Read the model definition and answer for the solid it produces. Units are mm, in the model's axes. A direction names the side the tool comes from. Give positions to 0.01 mm unless a question says otherwise; leave off trailing zeros. Loops run counter-clockwise (first coordinate to the right, second up) from the corner with the lowest first, then second, coordinate; pieces in that order, holes last.
(1) Straight lines are drawn through the part: probe 1 along Y at (x, z) = (0, -10.8); probe 2 along Y at (x, z) = (52, -10); probe 3 along Z at (x, y) = (-52.5, -42). For each, find the intervals that lie inside material, in ascending order.
(2) Each of these flat-tipped pins is pushed along its axis until it touches: P1, Ø13.5, axis at x = 0, y = -45, coming from the -Z side; P2, Ø10, axis at x = 28, y = -45, coming from the +Z side; P3, Ø6, axis at x = 28.5, z = -8.5, coming from the +Y side; P4, Ø6, axis at x = -22.5, y = -79, coming from the -Z side. Where does it stop, or does it pass through?
(3) Find section A-A, the plane y = -45. Write down the section's boundary in (x, z).
(4) Find section D-D, the plane y = 31.5. Write down the section's boundary in (x, z).
(5) Find section B-B, the plane x = 28. Write down the section's boundary in (y, z).
(6) Which of the six approach directions +Z, -Z, +X, -X, +Y, -Y give full straight-line access (tool end or side, diameter ignored) to faces 5 (the face through (1, -77, -3)), 6 (the face through (0.896, -59.542, -4.714)), 7 (the face through (32.246, 44.813, -10.979))?
(7) Determine the mould class of faces 1 (the face through (59.944, -83.49, -1.521)), 2 (the face through (-51.524, -80.797, -1.479)), 3 (the face through (-54.76, -27.73, -10.98)), 4 (the face through (1, 1, -12.5)) for opening direction X: pulls with the +X half, pulls with the -X half, needs draft (parallel to the pull), parting line crosses it, or undercut.
(8) Find section C-C, the plane y = -2. Write down the section's boundary in (x, z), then the cut area to 3 significant figures.
```python
from build123d import *

# Parameters (mm, degrees)
EXTRUDE_1_DEPTH     = 64
CHAMFER_1_SIZE      = 8
SKETCH_4_R          = 4.25
CUT_EXTRUDE_1_DEPTH = 110.073337851
SKETCH_6_R          = 4.25
CUT_EXTRUDE_2_DEPTH = 10


with BuildPart() as part:
    # 草图1 → 凸台-拉伸1 (new, symmetric)
    with BuildSketch(Plane(origin=(0, 0, 0), x_dir=(0, 0, -1), z_dir=(1, 0, 0))):
        with BuildLine():
            Line((0, 87.434221161), (3, 87.434221161))
            Line((3, 87.434221161), (3, 66.740486184))
            ThreePointArc((3, 66.740486184), (3.565077878, 64.198514208), (5.153873841, 62.135346276))
            Line((5.153873841, 62.135346276), (10.346126159, 57.798874885))
            ThreePointArc((10.346126159, 57.798874885), (11.934922122, 55.735706953), (12.5, 53.193734977))
            Line((12.5, 53.193734977), (12.5, -53.193734977))
            ThreePointArc((12.5, -53.193734977), (11.934922122, -55.735706953), (10.346126159, -57.798874885))
            Line((10.346126159, -57.798874885), (5.153873841, -62.135346276))
            ThreePointArc((5.153873841, -62.135346276), (3.565077878, -64.198514208), (3, -66.740486184))
            Line((3, -66.740486184), (3, -87.434221161))
            Line((3, -87.434221161), (0, -87.434221161))
            Line((0, -87.434221161), (0, -66.285275099))
            ThreePointArc((0, -66.285275099), (0.565077878, -63.743303123), (2.153873841, -61.680135191))
            Line((2.153873841, -61.680135191), (7.346126159, -57.3436638))
            ThreePointArc((7.346126159, -57.3436638), (8.934922122, -55.280495868), (9.5, -52.738523893))
            Line((9.5, -52.738523893), (9.5, 52.738523893))
            ThreePointArc((9.5, 52.738523893), (8.934922122, 55.280495868), (7.346126159, 57.3436638))
            Line((7.346126159, 57.3436638), (2.153873841, 61.680135191))
            ThreePointArc((2.153873841, 61.680135191), (0.565077878, 63.743303123), (0, 66.285275099))
            Line((0, 66.285275099), (0, 87.434221161))
        make_face()
    extrude(amount=EXTRUDE_1_DEPTH, both=True)

    # 倒角1
    chamfer_1_edges = [part.edges().sort_by_distance(p)[0] for p in [
        (-64, 87.434221161, -1.5),
        (-64, -87.434221161, -1.5),
        (64, -87.434221161, -1.5),
        (64, 87.434221161, -1.5),
    ]]
    chamfer(chamfer_1_edges, length=CHAMFER_1_SIZE)

    # 草图4 → 切除-拉伸1 (cut, through all)
    with BuildSketch(Plane.XY):
        with Locations((-52.800881805, 76.743624005)):
            Circle(SKETCH_4_R)
        with Locations((53.199118195, 76.743624005)):
            Circle(SKETCH_4_R)
        with Locations((-52.800881805, 31.5)):
            Circle(SKETCH_4_R)
        with Locations((-28, 45)):
            Circle(SKETCH_4_R)
        with Locations((0, 45)):
            Circle(SKETCH_4_R)
        with Locations(Location((52.800881805, 31.5, 0), (0, 0, 180))):
            Circle(SKETCH_4_R)
        with Locations(Location((28, 45, 0), (0, 0, 180))):
            Circle(SKETCH_4_R)
        with Locations(Location((53.199118195, -76.743624005, 0), (0, 0, 270))):
            Circle(SKETCH_4_R)
        with Locations((52.800881805, -31.5)):
            Circle(SKETCH_4_R)
        with Locations((28, -45)):
            Circle(SKETCH_4_R)
        with Locations(Location((0, -45, 0), (0, 0, 180))):
            Circle(SKETCH_4_R)
        with Locations(Location((-28, -45, 0), (0, 0, 180))):
            Circle(SKETCH_4_R)
        with Locations(Location((-52.800881805, -31.5, 0), (0, 0, 180))):
            Circle(SKETCH_4_R)
        with Locations(Location((-52.800881805, -76.743624005, 0), (0, 0, 270))):
            Circle(SKETCH_4_R)
    extrude(amount=-CUT_EXTRUDE_1_DEPTH, mode=Mode.SUBTRACT)

    # 草图6 → 切除-拉伸2 (cut)
    with BuildSketch(Plane(origin=(0, 0, -12.5), x_dir=(-1, 0, 0), z_dir=(0, 0, -1))):
        with Locations((-53, 0)):
            Circle(SKETCH_6_R)
        with Locations((53, 0)):
            Circle(SKETCH_6_R)
    extrude(amount=-CUT_EXTRUDE_2_DEPTH, mode=Mode.SUBTRACT)


solid = part.part
```
Entries:
1. probe 1: y = -57.38 to -49.25, -40.75 to 40.75, 49.25 to 57.38
1. probe 2: y = -58.09 to -35.67, -27.33 to -4.13, 4.13 to 27.33, 35.67 to 58.09
1. probe 3: z = -12.5 to -9.5
2. P1: stops at z = -12.5
2. P2: stops at z = -9.5
2. P3: stops at y = 61.85
2. P4: stops at z = -3
3. outline: (-64, -12.5) - (-32.25, -12.5) - (-32.25, -9.5) - (-64, -9.5) - close; (-23.75, -12.5) - (-4.25, -12.5) - (-4.25, -9.5) - (-23.75, -9.5) - close; (4.25, -12.5) - (23.75, -12.5) - (23.75, -9.5) - (4.25, -9.5) - close; (32.25, -12.5) - (64, -12.5) - (64, -9.5) - (32.25, -9.5) - close
4. outline: (-64, -12.5) - (-57.05, -12.5) - (-57.05, -9.5) - (-64, -9.5) - close; (-48.55, -12.5) - (48.55, -12.5) - (48.55, -9.5) - (-48.55, -9.5) - close; (57.05, -12.5) - (64, -12.5) - (64, -9.5) - (57.05, -9.5) - close
5. outline: (-87.43, -3) - (-66.74, -3) arc R6 cw to (-62.14, -5.15) - (-57.8, -10.35) arc R6 ccw to (-53.19, -12.5) - (-49.25, -12.5) - (-49.25, -9.5) - (-52.74, -9.5) arc R6 cw to (-57.34, -7.35) - (-61.68, -2.15) arc R6 ccw to (-66.29, 0) - (-87.43, 0) - close; (-40.75, -12.5) - (40.75, -12.5) - (40.75, -9.5) - (-40.75, -9.5) - close; (49.25, -12.5) - (53.19, -12.5) arc R6 ccw to (57.8, -10.35) - (62.14, -5.15) arc R6 cw to (66.74, -3) - (87.43, -3) - (87.43, 0) - (66.29, 0) arc R6 ccw to (61.68, -2.15) - (57.34, -7.35) arc R6 cw to (52.74, -9.5) - (49.25, -9.5) - close
6. face 5: -Z, +X, -X, -Y
6. face 6: +Z, +X, -X
6. face 7: +Z, -Z
7. face 1: pulls with the +X half
7. face 2: undercut
7. face 3: undercut
7. face 4: needs draft
8. outline: (-64, -12.5) - (-56.75, -12.5) - (-56.75, -9.5) - (-64, -9.5) - close; (-49.25, -12.5) - (49.25, -12.5) - (49.25, -9.5) - (-49.25, -9.5) - close; (56.75, -12.5) - (64, -12.5) - (64, -9.5) - (56.75, -9.5) - close
8. area: 339 mm2
